Geometry: final body of the model. Coordinates: model frame, mm. Round coordinates to 2 decimals unless told otherwise and drop trailing zeros. Order: outer loops, then holes, each group sorted by start corner. A loop starts at its lowest first (then second) coordinate and runs counter-clockwise, first axis right, second up. Notation, with made-up numbers: M 28.25,-26.75 L 53.25,-26.75 A28 cw 53.25,-3.75 Z; hole C 62,-29.5 d6. An arc over 180 degrees is marked long. Put each result on its own line as item: value. Start each with the question number.
1) Material intervals for probe 1 along X at (y, z) = (-2, 207.5); probe 2 along Y at (x, z) = (6, 614.5); probe 3 along Z at (x, y) = (0, 6.8), sorted ascending. Write a range as [from, to].
2) First-contact query: P1, Ø1.5, axis at x = 5, y = -1, coming from the -Z side. Flat tip, straight axial feed; report the tip coordinate or a pass-through.
3) Section A-A, the plane z = 731. Return loops of the section in (x, y).
from build123d import *

# Parameters (mm, degrees)
EXTRUDE1_DEPTH     = 1000
SKETCH2_R          = 2
CUT_EXTRUDE1_DEPTH = 2
SKETCH3_R          = 2
CUT_EXTRUDE2_DEPTH = 2


with BuildPart() as part:
    # Sketch1 → Extrude1 (new body)
    with BuildSketch(Plane.XY):
        with BuildLine():
            Line((-5.8, 7.5), (5.8, 7.5))
            ThreePointArc((5.8, 7.5), (7.002081528, 7.002081528), (7.5, 5.8))
            Line((7.5, 5.8), (7.5, -5.8))
            ThreePointArc((7.5, -5.8), (7.002081528, -7.002081528), (5.8, -7.5))
            Line((5.8, -7.5), (-5.8, -7.5))
            ThreePointArc((-5.8, -7.5), (-7.002081528, -7.002081528), (-7.5, -5.8))
            Line((-7.5, -5.8), (-7.5, 5.8))
            ThreePointArc((-7.5, 5.8), (-7.002081528, 7.002081528), (-5.8, 7.5))
        make_face()
        with BuildLine():
            Line((-6.3, 5.8), (-6.3, -5.8))
            ThreePointArc((-6.3, -5.8), (-6.153553391, -6.153553391), (-5.8, -6.3))
            Line((-5.8, -6.3), (5.8, -6.3))
            ThreePointArc((5.8, -6.3), (6.153553391, -6.153553391), (6.3, -5.8))
            Line((6.3, -5.8), (6.3, 5.8))
            ThreePointArc((6.3, 5.8), (6.153553391, 6.153553391), (5.8, 6.3))
            Line((5.8, 6.3), (-5.8, 6.3))
            ThreePointArc((-5.8, 6.3), (-6.153553391, 6.153553391), (-6.3, 5.8))
        make_face(mode=Mode.SUBTRACT)
    extrude(amount=EXTRUDE1_DEPTH)

    # Sketch2 → Cut-Extrude1 (cut)
    with BuildSketch(Plane.ZY.offset(7.5)):
        with Locations((697, 0)):
            Circle(SKETCH2_R)
    extrude(amount=-CUT_EXTRUDE1_DEPTH, mode=Mode.SUBTRACT)

    # Sketch3 → Cut-Extrude2 (cut)
    with BuildSketch(Plane(origin=(0, 7.5, 0), x_dir=(-1, 0, 0), z_dir=(0, 1, 0))):
        with Locations((0, 650)):
            Circle(SKETCH3_R)
    extrude(amount=-CUT_EXTRUDE2_DEPTH, mode=Mode.SUBTRACT)


solid = part.part
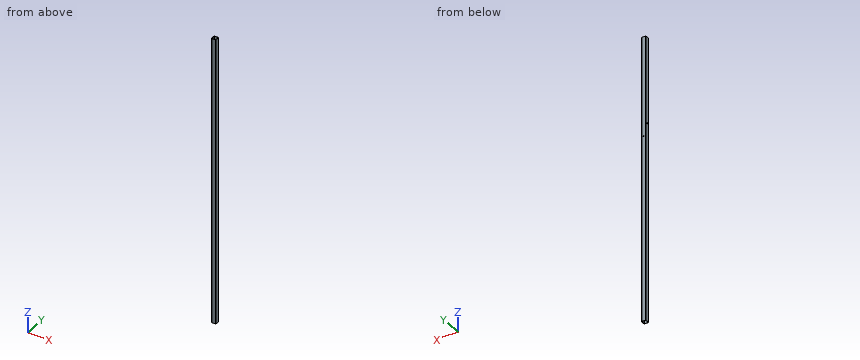
Result sheet:
1. probe 1: x = [-7.5, -6.3], [6.3, 7.5]
1. probe 2: y = [-7.49, -6.26], [6.26, 7.49]
1. probe 3: z = [0, 648], [652, 1000]
2. P1: passes through
3. outline: M -7.5,-5.8 A1.7 ccw -5.8,-7.5 L 5.8,-7.5 A1.7 ccw 7.5,-5.8 L 7.5,5.8 A1.7 ccw 5.8,7.5 L -5.8,7.5 A1.7 ccw -7.5,5.8 Z; hole M -6.3,-5.8 A0.5 ccw -5.8,-6.3 L 5.8,-6.3 A0.5 ccw 6.3,-5.8 L 6.3,5.8 A0.5 ccw 5.8,6.3 L -5.8,6.3 A0.5 ccw -6.3,5.8 Z
